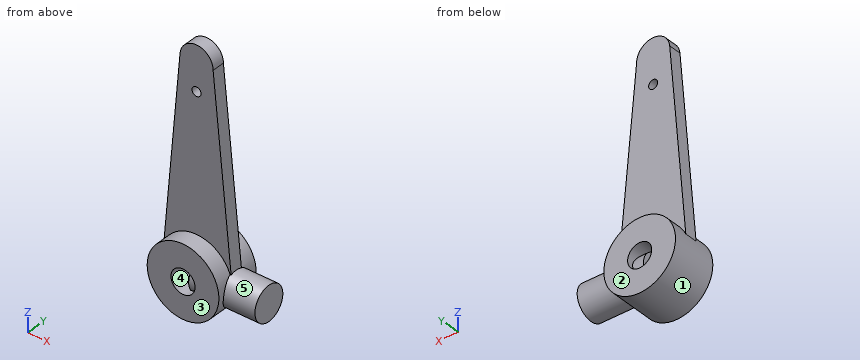
Autodesk Inventor part; units mm, degrees
ref_plane "Work Plane1" through (-0.1567, -1.05, 63.0829) normal (1, 0, 0.0049) x (0, 1, 0)
ref_plane "YZ Plane" through (0, 0, 0) normal (1, 0, 0) x (0, 1, 0)
ref_plane "XZ Plane" through (0, 0, 0) normal (0, 1, 0) x (-1, 0, 0)
sketch "Sketch1" plane through (0, 0, 0) normal (0, 1, 0) x (-1, 0, 0)
  circle A0 centre (0, 0) radius 5.95
  line L0 (0, 0) -> (0, 33.07)
  circle A1 centre (0, 33.07) radius 2.75
  line L1 (5.4153, 2.4652) -> (2.7393, 33.3118)
  line L2 (-5.8278, 1.1997) -> (-2.7497, 33.029)
  dimension "d0" = 11.9
  dimension "d1" = 5.5
  dimension "d2" = 33.07
extrude "Extrusion1" add sketch "Sketch1" along normal mid plane 7.63 contours A0
extrude "Extrusion2" add sketch "Sketch1" along normal mid plane 2.1 contours A0 L0 A1 L1 | L2 A1 L0 A0 | A1
sketch "Sketch2" plane through (0, 1.05, 0) normal (0, 1, 0) x (1, 0, 0)
  arc A0 (-2.7393, -33.3118) -> (2.7497, -33.029) centre (0, -33.07) ccw construction
  line L0 (0, -35.82) -> (0, -28.45) construction
  circle A1 centre (0, -28.45) radius 0.75
  point P0 (0, 0)
  dimension "d7" = 7.37
  dimension "d8" = 1.5
extrude "Extrusion3" cut sketch "Sketch2" against normal blind 2.1
sketch "Sketch3" plane through (0, 3.815, 0) normal (0, 1, 0) x (1, 0, 0)
  circle A0 centre (0, 0) radius 2
  point P0 (0, 0)
  dimension "d11" = 4
extrude "Extrusion4" cut sketch "Sketch3" against normal blind 50
ref_plane "Work Plane1" through (-0.1567, -1.05, 63.0829) normal (1, 0, 0.0049) x (0, 1, 0)
sketch "Sketch4" plane through (-0.1567, -1.05, 63.0829) normal (1, 0, 0.0049) x (0, 1, 0)
  circle A0 centre (1.05, -63.6808) radius 2.85
  point P0 (1.05, -63.0829)
  dimension "d14" = 5.7
extrude "Extrusion5" add sketch "Sketch4" along normal blind 11
properties part number "Nose Gear Steering Arm"
Here's how the part is built. I have some questions about the finished solid (model axes, mm). Face numbers are marked on the shaded views. A direction names the side the tool comes from. Coordinates: 2 decimals unless noted, no trailing zeros. Write each loop counter-clockwise with the first axis right and the second up, starting at its lowest first coordinate (ties: lowest second). Pieces come first, ordered by that corner, then holes. Notation, with made-up numbers: (48, -22.75) - (106, -22.75) arc R14 cw to (106, -6.75) - close; hole circle Ø5 at (46, 9). An arc over 180 degrees is marked (long way). One line per item, written item: value.
1) Suppose I cut it at B-B on z = 10. Write out the boundary of the cut face in (x, y), and give its area (3 significant figures).
Model answer:
outline: (-4.76, -1.05) - (4.98, -1.05) - (4.98, 1.05) - (-4.76, 1.05) - close
area: 20.5 mm²
2) I'm going to push flat-ended pins straight in: P1, Ø4, axis at x = -4, y = -2, coming from the -Z side; P2, Ø2, axis at x = 0, z = 28.45, coming from the +Y side; P3, Ø1, axis at x = -3.5, y = 1.5, coming from the -Z side. Where does each tip first touch, or does it pass through?
Model answer:
P1: stops at z = -5.6
P2: stops at y = 1.05
P3: stops at z = -5.14
3) I need wall thicknesses on line 1 along Z through (x, y) = (0, 0.25); line 2 along X through (y, z) = (-1.75, 0); line 3 along X through (y, z) = (0.05, 28.45). Which ranges of each line are inside material? Lowest first, please.
Model answer:
line 1: z = -5.95 to -2, 2 to 27.7, 29.2 to 35.82
line 2: x = -5.95 to -2, 0.15 to 11.15
line 3: x = -3.16 to -0.75, 0.75 to 3.19
4) On a 3-axis mill with a long thin cutter (end or side, diameter ignored), from which of +Z, -Z, +X, -X, +Y, -Y can I reach the whole of each face in a straight line? I mean the marked faces 1 and 2. Say none if no direction works.
Model answer:
face 1: none
face 2: +Z, -Z, +X, -X, +Y
5) Suppose I cut it at C-C on z = 24. Write out the boundary of the cut face in (x, y).
Model answer:
outline: (-3.55, -1.05) - (3.62, -1.05) - (3.62, 1.05) - (-3.55, 1.05) - close
6) Suppose I cut it at A-A on z = 28.45. Write out the boundary of the cut face in (x, y), and give its area (3 significant figures).
Model answer:
outline: (-3.16, -1.05) - (-0.75, -1.05) - (-0.75, 1.05) - (-3.16, 1.05) - close; (0.75, -1.05) - (3.19, -1.05) - (3.19, 1.05) - (0.75, 1.05) - close
area: 10.2 mm²
7) We'd pull the mould along Z, two halves only. Please class the marked faces 3, 4 and 5: pulls with the +Z half, pulls with the -Z half, needs draft (parallel to the pull), parting line crosses it, or undercut.
Model answer:
face 3: needs draft
face 4: undercut
face 5: parting line crosses it
